from build123d import *

# Parameters (mm, degrees)
SKETCH1_W                       = 812.8
SKETCH1_H                       = 77.724
BOSS_EXTRUDE1_DEPTH             = 19.05
SKETCH2_W                       = 71.374
SKETCH2_H                       = 15.875
CUT_EXTRUDE1_DEPTH              = 817.296745672
CUT_EXTRUDE2_REACH              = 818.662
SKETCH3_W                       = 762
SKETCH3_H                       = 11.1125
HOLE1_D                         = 28.575
HOLE1_DEPTH                     = 19.05
HOLE2_D                         = 9.652
HOLE2_DEPTH                     = 19.05
F_2_CLEARANCE_HOLE1_D           = 2.54
F_2_CLEARANCE_HOLE1_DEPTH       = 19.05
F_3_4_0_75_DIAMETER_HOLE1_D     = 19.05
F_3_4_0_75_DIAMETER_HOLE1_DEPTH = 19.05
F_1_4_CLEARANCE_HOLE1_D         = 6.7056
F_1_4_CLEARANCE_HOLE1_DEPTH     = 19.05
F_10_CLEARANCE_HOLE1_D          = 5.334
F_10_CLEARANCE_HOLE1_DEPTH      = 3.175
F_10_CLEARANCE_HOLE2_D          = 5.334
F_10_CLEARANCE_HOLE2_DEPTH      = 77.724
CHAMFER1_SIZE                   = 3.175
FILLET1_R                       = 0.762
FILLET2_R                       = 3.937


with BuildPart() as part:
    # Sketch1 → Boss-Extrude1 (new body)
    with BuildSketch(Plane.XZ.offset(15.875)):
        with Locations((406.4, -34.925)):
            Rectangle(SKETCH1_W, SKETCH1_H)
    extrude(amount=-BOSS_EXTRUDE1_DEPTH)

    # Sketch2 → Cut-Extrude1 (cut, through all)
    with BuildSketch(Plane.ZY):
        with Locations((-34.925, -7.9375)):
            Rectangle(SKETCH2_W, SKETCH2_H)
    extrude(amount=-CUT_EXTRUDE1_DEPTH, mode=Mode.SUBTRACT)

    # Sketch3 → Cut-Extrude2 (cut, up to next)
    with BuildSketch(Plane.XY.offset(3.937), mode=Mode.PRIVATE) as cut_extrude2_sk1:
        with Locations((406.4, -10.31875)):
            Rectangle(SKETCH3_W, SKETCH3_H)
    cut_extrude2_tool1 = extrude(cut_extrude2_sk1.sketch, amount=-CUT_EXTRUDE2_REACH, mode=Mode.PRIVATE) & part.part
    add(cut_extrude2_tool1.solids().sort_by_distance((406.4, -10.31875, 3.937))[0], mode=Mode.SUBTRACT)

    # Hole1
    with Locations(Plane(origin=(0, 3.175, 0), x_dir=(1, 0, 0), z_dir=(0, 1, 0))):
        with Locations((406.4, 17.272)):
            Hole(HOLE1_D / 2, depth=HOLE1_DEPTH)

    # Hole2
    with Locations(Plane(origin=(0, 3.175, 0), x_dir=(1, 0, 0), z_dir=(0, 1, 0))):
        with Locations((568.924874752, 19.05), (601.438495912, 19.05), (628.947697627, 19.05), (243.875125248, 19.05), (211.361504088, 19.05), (183.852302373, 19.05), (678.944202666, 20.828), (701.450372003, 20.828), (726.460886343, 20.828), (133.855797334, 20.828), (111.349627997, 20.828), (86.339113657, 20.828)):
            Hole(HOLE2_D / 2, depth=HOLE2_DEPTH)

    # #2 Clearance Hole1
    with Locations(Plane(origin=(0, 3.175, 0), x_dir=(1, 0, 0), z_dir=(0, 1, 0))):
        with Locations((711.2, 3.175), (711.2, 66.675), (762, 3.175), (762, 66.675), (101.6, 3.175), (50.8, 3.175), (101.6, 66.675), (50.8, 66.675)):
            Hole(F_2_CLEARANCE_HOLE1_D / 2, depth=F_2_CLEARANCE_HOLE1_DEPTH)

    # 3/4 (0.75) Diameter Hole1
    with Locations(Plane(origin=(0, 3.175, 0), x_dir=(1, 0, 0), z_dir=(0, 1, 0))):
        with Locations((690.197287335, 33.02), (642.712889143, 33.02), (170.087110857, 33.02), (122.602712665, 33.02)):
            Hole(F_3_4_0_75_DIAMETER_HOLE1_D / 2, depth=F_3_4_0_75_DIAMETER_HOLE1_DEPTH)

    # 1/4 Clearance Hole1
    with Locations(Plane(origin=(0, 3.175, 0), x_dir=(1, 0, 0), z_dir=(0, 1, 0))):
        with Locations((641.35, 14.732), (546.1, 14.732), (171.45, 14.732), (266.7, 14.732), (513.925467617, 17.547282407), (298.874532383, 17.547282407)):
            Hole(F_1_4_CLEARANCE_HOLE1_D / 2, depth=F_1_4_CLEARANCE_HOLE1_DEPTH)

    # #10 Clearance Hole1
    with Locations(Plane(origin=(0, 0, 0.762), x_dir=(-1, 0, 0), z_dir=(0, 0, -1))):
        with Locations((-12.7, -9.525), (-800.1, -9.525)):
            Hole(F_10_CLEARANCE_HOLE1_D / 2, depth=F_10_CLEARANCE_HOLE1_DEPTH)

    # #10 Clearance Hole2
    with Locations(Plane(origin=(0, 0, -73.787), x_dir=(-1, 0, 0), z_dir=(0, 0, -1))):
        with Locations((-800.1, -9.525), (-774.7, -9.525), (-749.3, -9.525), (-723.9, -9.525), (-698.5, -9.525), (-673.1, -9.525), (-647.7, -9.525), (-622.3, -9.525), (-596.9, -9.525), (-571.5, -9.525), (-546.1, -9.525), (-520.7, -9.525), (-495.3, -9.525), (-469.9, -9.525), (-444.5, -9.525), (-419.1, -9.525), (-393.7, -9.525), (-368.3, -9.525), (-342.9, -9.525), (-317.5, -9.525), (-292.1, -9.525), (-266.7, -9.525), (-241.3, -9.525), (-215.9, -9.525), (-190.5, -9.525), (-165.1, -9.525), (-139.7, -9.525), (-114.3, -9.525), (-88.9, -9.525), (-63.5, -9.525), (-38.1, -9.525), (-12.7, -9.525)):
            Hole(F_10_CLEARANCE_HOLE2_D / 2, depth=F_10_CLEARANCE_HOLE2_DEPTH)

    # Chamfer1
    chamfer1_edges = [part.edges().sort_by_distance(p)[0] for p in [
        (812.8, -15.875, 2.3495),
        (0, -15.875, -72.1995),
        (787.4, -4.7625, 2.3495),
        (25.4, -4.7625, 2.3495),
        (25.4, -15.875, 2.3495),
        (787.4, -15.875, 2.3495),
        (0, -15.875, 2.3495),
        (812.8, -15.875, -72.1995),
    ]]
    chamfer(chamfer1_edges, length=CHAMFER1_SIZE)

    # Fillet1
    fillet1_edges = [part.edges().sort_by_distance(p)[0] for p in [
        (406.4, 0, -70.612),
        (406.4, 0, 0.762),
    ]]
    fillet(fillet1_edges, radius=FILLET1_R)

    # Fillet2
    fillet2_edges = [part.edges().sort_by_distance(p)[0] for p in [
        (406.4, 3.175, -73.787),
        (406.4, 3.175, 3.937),
    ]]
    fillet(fillet2_edges, radius=FILLET2_R)


solid = part.part
Read the model definition and answer for the solid it produces. Units are mm, in the model's axes. A direction names the side the tool comes from. Give positions to 0.01 mm unless a question says otherwise; leave off trailing zeros. Write each loop counter-clockwise with the first axis right and the second up, starting at its lowest first coordinate (ties: lowest second). Pieces come first, ordered by that corner, then holes. Notation, with made-up numbers: (10.25, 39.25) - (66.25, 39.25) arc R17 ccw to (66.25, 60.25) - close; hole circle Ø1 at (2.5, 6.25). An arc over 180 degrees is marked (long way). Use CSV: the item, a comma, the result in double quotes. Start each with the question number.
Item 1: The part is cut by section A-A, the plane z = -51. Give the vertices of the cut face in (x, y) (3 decimals).
Item 2: The mould has two halves that part along Z. Classify faces 3 (the flat face through (465, -3, 0.762)), 4 (the flat face through (401, 3.175, -34)), 5 (the flat face through (405, -4, 3.937)), 6 (the cylindrical face through (699.713, 1.565, -33.439)): pulls with the +Z half, pulls with the -Z half, needs draft (parallel to the pull), parting line crosses it, or undercut.
Item 3: For faces 1 (the cylindrical face through (161.29, 1.57, -29.37)), 2 (the flat face through (401, -8, -70.612)), determine the directions among +Z, -Z, +X, -X, +Y, -Y from which every point of the face is accessible in a straight line to the end or side of a thin tool.
Item 4: Flat-ended cylindrical pins translate along their axes: P1, Ø15.5, axis at x = 701.45, z = -20.83, coming from the -Y side; P2, Ø4, axis at x = 121, y = -8.5, coming from the +Z side; P3, Ø1.5, axis at x = 253.5, y = 1, coming from the -Z side. Find the tip coordinate at first contact, or state that the pin passes through.
Item 5: Consider line 1 (Z direction, x = 101, y = 0.25); line 2 (Z direction, x = 136.5, y = -3.5); line 3 (Z direction, x = 134.5, y = -7). Determine where each line is inside the solid, lowest interval first.
Taken from the geometry:
1,outline,"(0, 0) - (812.8, 0) - (812.8, 3.175) - (0, 3.175) - close"
2,face 3,"undercut"
2,face 4,"needs draft"
2,face 5,"pulls with the +Z half"
2,face 6,"undercut"
3,face 1,"+Y, -Y"
3,face 2,"+X, -X, -Y"
4,P1,"y = 0"
4,P2,"z = -70.61"
4,P3,"z = -73.65"
5,line 1,"-73.65 to -67.79, -65.56 to -4.29, -2.06 to 3.8"
5,line 2,"-73.79 to -70.61, 0.76 to 3.94"
5,line 3,"-73.79 to -70.61"
